For this review, take the finished solid that the model builds, in its own axes (mm). Face numbers are marked on the shaded views. Round coordinates to 2 decimals unless told otherwise and drop trailing zeros. Order: outer loops, then holes, each group sorted by start corner. A loop starts at its lowest first (then second) coordinate and runs counter-clockwise, first axis right, second up. Notation, with made-up numbers: (-13.5, 50) - (18.5, 50) arc R17 cw to (18.5, 77) - close; hole circle Ø6 at (-37.5, 41). An arc over 180 degrees is marked (long way). Write each question's results on one line, items separated by ' | '. Start each with the question number.
(1) For L1, parallel to Z at x = -6.5, y = -23.5; L2, parallel to Z at x = 3, y = -18; L3, parallel to X at y = -2, z = 7, list the stretches that pass through material, from the lowest coordinate up. Write a range as from..to.
(2) Take a section at B-B, the plane z = 6. Give the boundary of the cut face in (x, y), plus the area to 3 significant figures.
(3) Take a section at C-C, the plane x = 0. Give the boundary of the cut face in (y, z).
(4) Take a section at D-D, the plane z = 20.5. Give the boundary of the cut face in (x, y), plus the area to 3 significant figures.
(5) Draft analysis for pull direction X (two halves, no side actions). For the marked faces 1, 2, 3 and 4, state which applies: pulls with the +X half, pulls with the -X half, needs draft (parallel to the pull), parting line crosses it, or undercut.
(6) Insertion check: pin 1 Ø6 at (x, y) = (5.5, -4) entering from -Z; pin 2 Ø10 at (x, y) = (11, -11.5) entering from +Z; pin 3 Ø10 at (y, z) = (-13.5, 22) entering from +X. Each pin has a flat end and moves straight along its axis. Give the tip position at first contact, or say it passes through.
(7) Take a section at A-A, the plane y = -7.25. Give the boundary of the cut face in (x, z), plus the area to 3 significant figures.
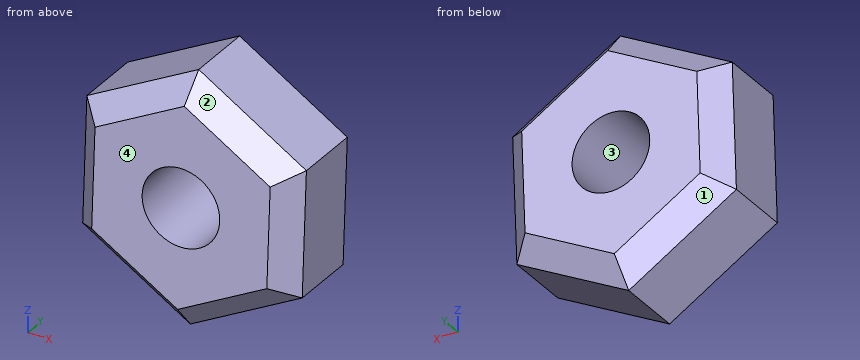
```python
from build123d import *

# Parameters (mm, degrees)
F1_DEPTH = 25.4
F2_SIZE  = 5.08
F3_SIZE  = 5.08
F5_D     = 17.78


with BuildPart() as f1:
    # F0 (on Front) → F1 (new body)
    with BuildSketch(Plane.XZ):
        Polygon((25.60047, 13.673016), (0.959056, 29.007166), (-24.641414, 15.33415), (-25.60047, -13.673016), (-0.959056, -29.007166), (24.641414, -15.33415), align=None)
    extrude(amount=F1_DEPTH)

    # F2
    f2_edges = [f1.edges().sort_by_distance(p)[0] for p in [
        (13.279763, -25.4, 21.340091),
        (25.120942, -25.4, -0.830567),
        (11.841179, -25.4, -22.170658),
        (-13.279763, -25.4, -21.340091),
        (-25.120942, -25.4, 0.830567),
        (-11.841179, -25.4, 22.170658),
    ]]
    chamfer(f2_edges, length=F2_SIZE)

    # F3
    f3_edges = [f1.edges().sort_by_distance(p)[0] for p in [
        (25.120942, 0, -0.830567),
        (13.279763, 0, 21.340091),
        (11.841179, 0, -22.170658),
        (-11.841179, 0, 22.170658),
        (-25.120942, 0, 0.830567),
        (-13.279763, 0, -21.340091),
    ]]
    chamfer(f3_edges, length=F3_SIZE)

    # F5 (through all)
    with Locations(Plane.XZ.offset(25.4)):
        with Locations((0, 0)):
            Hole(F5_D / 2)


solid = f1.part
```
Results below:
1) L1: z = -21.81..-6.06, 6.06..21.42 | L2: z = -26.89..-8.37, 8.37..27.74 | L3: x = -21.84..-5.48, 5.48..22.3
2) outline: (-24.95, -20.32) - (-19.87, -25.4) - (-6.56, -25.4) - (-6.56, 0) - (-19.87, 0) - (-24.95, -5.08) - close; (6.56, -25.4) - (20.26, -25.4) - (25.35, -20.32) - (25.35, -5.08) - (20.26, 0) - (6.56, 0) - close | area: 893 mm^2
3) outline: (-25.4, -22.74) - (-20.32, -28.49) - (-5.08, -28.49) - (0, -22.74) - (0, -8.89) - (-25.4, -8.89) - close; (-25.4, 8.89) - (0, 8.89) - (0, 22.74) - (-5.08, 28.49) - (-20.32, 28.49) - (-25.4, 22.74) - close
4) outline: (-14.97, -20.32) - (-4.19, -25.4) - (5.01, -25.4) - (14.63, -20.32) - (14.63, -5.08) - (5.01, 0) - (-4.19, 0) - (-14.97, -5.08) - close | area: 648 mm^2
5) face 1: pulls with the -X half | face 2: pulls with the +X half | face 3: undercut | face 4: needs draft
6) pin 1: stops at z = -27.05 | pin 2: stops at z = 25.87 | pin 3: stops at x = 20.25
7) outline: (-25.6, -13.67) - (-0.96, -29.01) - (24.64, -15.33) - (25.6, 13.67) - (0.96, 29.01) - (-24.64, 15.33) - close; hole circle Ø17.78 at (0, 0) | area: 1,940 mm^2
